from build123d import *

# Parameters (mm, degrees)
SKETCH1_R           = 12.1
BOSS_EXTRUDE1_DEPTH = 30.5
CUT_EXTRUDE1_DEPTH  = 40.56096561


with BuildPart() as part:
    # Sketch1 → Boss-Extrude1 (new body)
    with BuildSketch(Plane.XY):
        with Locations(Location((0, 0, 0), (0, 0, 180))):
            Circle(SKETCH1_R)
    extrude(amount=BOSS_EXTRUDE1_DEPTH)

    # Sketch2 → Cut-Extrude1 (cut, through all)
    with BuildSketch(Plane(origin=(0, 10, 0), x_dir=(1, 0, 0), z_dir=(0, 1, 0))):
        Polygon((-2, -9.569188556), (-4.8, -9.569188556), (-4.8, -14.104311921), (-2, -19.069188556), align=None)
        Polygon((4.8, -14.104311921), (2, -19.069188556), (2, -9.569188556), (4.8, -9.569188556), align=None)
    extrude(amount=CUT_EXTRUDE1_DEPTH, mode=Mode.SUBTRACT)


solid = part.part
Geometry: final body of the model. Coordinates: model frame, mm. A direction names the side the tool comes from. Give positions to 0.01 mm unless a question says otherwise; leave off trailing zeros. Write each loop counter-clockwise with the first axis right and the second up, starting at its lowest first coordinate (ties: lowest second). Pieces come first, ordered by that corner, then holes.
(1) Cut plane C-C, the plane y = -6. Return loops of the section in (x, z).
(2) Cut plane D-D, the plane z = 17. Return loops of the section in (x, y).
(3) Access query for faces 1 (the flat face through (3, 10, 13)), 2 (the cylindrical face through (-6.505, -10.203, 15.036)). Directions: +Z, -Z, +X, -X, +Y, -Y. A direction counts if a zero-diameter tool reaches every point of the face in a straight line with its end or side. Return the directions, or none.
(4) Cut plane A-A, the plane z = 24.5. Return loops of the section in (x, y), then the cut area to 3 significant figures.
(5) Mould query, pull axis Z, two halves, no side actions, for faces 3 (the flat face through (-4.8, 10.5, 11.8)), 4 (the flat face through (0, 0, 30.5)), 5 (the flat face through (0, 0, 0)). Classes: released by +Z, released by -Z, zero draft, split by the parting line, or undercut.
(6) Ray query, line 1 (X direction, y = 7.25, z = 24); line 2 (X direction, y = 9, z = 24); line 3 (Y direction, x = 7.5, z = 16.5). Return the intervals inside material, ascending.
(7) Cut plane B-B, the plane x = -3.75. Return loops of the section in (y, z), then the cut area to 3 significant figures.
(8) First-contact query: P1, Ø1.5, axis at y = 10.5, z = 16, coming from the -X side; P2, Ø0.8, axis at x = 4, z = 15.5, coming from the +Y side; P3, Ø4, axis at x = -5, y = -6.5, coming from the -Z side; P4, Ø1.5, axis at x = -7, z = 18.5, coming from the +Y side. Flat tips, straight axial feed; report the tip coordinate or a pass-through.
Values follow:
1. outline: (-10.51, 0) - (10.51, 0) - (10.51, 30.5) - (-10.51, 30.5) - close
2. outline: (-3.17, 10) - (-3.17, 11.68) arc R12.1 ccw (long way) to (3.17, 11.68) - (3.17, 10) - (2, 10) - (2, 11.93) arc R12.1 ccw to (-2, 11.93) - (-2, 10) - close
3. face 1: +Y
3. face 2: +Z, -Z
4. outline: circle Ø24.2 at (0, 0)
4. area: 460 mm2
5. face 3: undercut
5. face 4: released by +Z
5. face 5: released by -Z
6. line 1: x = -9.69 to 9.69
6. line 2: x = -8.09 to 8.09
6. line 3: y = -9.5 to 9.5
7. outline: (-11.5, 0) - (11.5, 0) - (11.5, 9.57) - (10, 9.57) - (10, 15.97) - (11.5, 15.97) - (11.5, 30.5) - (-11.5, 30.5) - close
7. area: 692 mm2
8. P1: stops at x = -7.17
8. P2: stops at y = 11.48
8. P3: stops at z = 0
8. P4: stops at y = 10.36
